from build123d import *

# Parameters (mm, degrees)
BOSS_EXTRUDE4_DEPTH = 5
SKETCH6_W           = 70
SKETCH6_H           = 70
BOSS_EXTRUDE5_DEPTH = 30
SKETCH8_R           = 3
CUT_EXTRUDE1_DEPTH  = 2
FILLET1_R           = 10
CUT_EXTRUDE2_DEPTH  = 30
BOSS_EXTRUDE6_DEPTH = 2.5
SKETCH11_W          = 2.5
SKETCH11_H          = 65
BOSS_EXTRUDE7_DEPTH = 27.5
FILLET2_R           = 10
CHAMFER1_SIZE       = 1.25
CHAMFER2_SIZE       = 1.25


with BuildPart() as part:
    # Sketch5 → Boss-Extrude4 (new body)
    with BuildSketch(Plane(origin=(0, 0, 0), x_dir=(1, 0, 0), z_dir=(0, 1, 0))):
        with BuildLine():
            Line((-22.5, -32.5), (22.5, -32.5))
            ThreePointArc((22.5, -32.5), (29.571067812, -29.571067812), (32.5, -22.5))
            Line((32.5, -22.5), (32.5, 22.5))
            ThreePointArc((32.5, 22.5), (29.571067812, 29.571067812), (22.5, 32.5))
            Line((22.5, 32.5), (-22.5, 32.5))
            ThreePointArc((-22.5, 32.5), (-29.571067812, 29.571067812), (-32.5, 22.5))
            Line((-32.5, 22.5), (-32.5, -22.5))
            ThreePointArc((-32.5, -22.5), (-29.571067812, -29.571067812), (-22.5, -32.5))
        make_face()
    extrude(amount=BOSS_EXTRUDE4_DEPTH)

    # Sketch6 → Boss-Extrude5 (add)
    with BuildSketch(Plane(origin=(0, 5, 0), x_dir=(1, 0, 0), z_dir=(0, 1, 0))):
        Rectangle(SKETCH6_W, SKETCH6_H)
    extrude(amount=BOSS_EXTRUDE5_DEPTH)

    # Sketch8 → Cut-Extrude1 (cut)
    with BuildSketch(Plane.XZ):
        with Locations(Location((26.037533906, -26.035533906, 0), (0, 0, 270))):
            Circle(SKETCH8_R)
        with Locations(Location((26.036533906, 26.036533906, 0), (0, 0, 270))):
            Circle(SKETCH8_R)
        with BuildLine():
            ThreePointArc((-23.035533906, 26.035533906), (-24.887483609, 28.807172503), (-28.156854249, 28.156854249))
            Line((-28.156854249, 28.156854249), (-23.914213562, 23.914213562))
            ThreePointArc((-23.914213562, 23.914213562), (-23.263895308, 24.887483609), (-23.035533906, 26.035533906))
        make_face()
        with BuildLine():
            Line((-23.914213562, 23.914213562), (-28.156854249, 28.156854249))
            ThreePointArc((-28.156854249, 28.156854249), (-28.156854249, 23.914213562), (-23.914213562, 23.914213562))
        make_face()
        with Locations(Location((-26.034533906, -26.036533906, 0), (0, 0, 270))):
            Circle(SKETCH8_R)
    extrude(amount=-CUT_EXTRUDE1_DEPTH, mode=Mode.SUBTRACT)

    # Fillet1
    fillet1_edges = [part.edges().sort_by_distance(p)[0] for p in [
        (-35, 20, -35),
        (-35, 20, 35),
        (35, 20, 35),
        (35, 20, -35),
    ]]
    fillet(fillet1_edges, radius=FILLET1_R)

    # Sketch9 → Cut-Extrude2 (cut)
    with BuildSketch(Plane(origin=(0, 35, 0), x_dir=(1, 0, 0), z_dir=(0, 1, 0))):
        with BuildLine():
            Line((25, 32.5), (-25, 32.5))
            ThreePointArc((-25, 32.5), (-30.303300859, 30.303300859), (-32.5, 25))
            Line((-32.5, 25), (-32.5, -25))
            ThreePointArc((-32.5, -25), (-30.303300859, -30.303300859), (-25, -32.5))
            Line((-25, -32.5), (25, -32.5))
            ThreePointArc((25, -32.5), (30.303300859, -30.303300859), (32.5, -25))
            Line((32.5, -25), (32.5, 25))
            ThreePointArc((32.5, 25), (30.303300859, 30.303300859), (25, 32.5))
        make_face()
    extrude(amount=-CUT_EXTRUDE2_DEPTH, mode=Mode.SUBTRACT)


with BuildPart() as cut_extrude2_piece_1:
    # of the separate pieces the step leaves, piece 1, a body of its own (cut_extrude2_pieces)
    add(part.part.solids().sort_by_distance((-22.5, 0, 32.5))[0])



with BuildPart() as cut_extrude2_piece_2:
    # of the separate pieces the step leaves, piece 2, a body of its own (cut_extrude2_pieces)
    add(part.part.solids().sort_by_distance((25, 5, -35))[0])


with BuildPart() as cut_extrude2_piece_1_1:
    add(cut_extrude2_piece_1.part)

    add(cut_extrude2_piece_2.part)  # Boss-Extrude6 merges Cut-Extrude2 piece 2
    # Sketch10 → Boss-Extrude6 (add)
    with BuildSketch(Plane.XZ.offset(-5)):
        with BuildLine():
            Line((-35, 25), (-35, -25))
            ThreePointArc((-35, -25), (-32.071067812, -32.071067812), (-25, -35))
            Line((-25, -35), (25, -35))
            ThreePointArc((25, -35), (32.071067812, -32.071067812), (35, -25))
            Line((35, -25), (35, 25))
            ThreePointArc((35, 25), (32.071067812, 32.071067812), (25, 35))
            Line((25, 35), (-25, 35))
            ThreePointArc((-25, 35), (-32.071067812, 32.071067812), (-35, 25))
        make_face()
    extrude(amount=-BOSS_EXTRUDE6_DEPTH)

    # Sketch11 → Boss-Extrude7 (add)
    with BuildSketch(Plane(origin=(0, 35, 0), x_dir=(1, 0, 0), z_dir=(0, 1, 0))):
        Rectangle(SKETCH11_W, SKETCH11_H)
    extrude(amount=-BOSS_EXTRUDE7_DEPTH)

    # Fillet2
    fillet2_edges = [cut_extrude2_piece_1_1.edges().sort_by_distance(p)[0] for p in [
        (-1.25, 21.25, -32.5),
        (-1.25, 21.25, 32.5),
        (1.25, 21.25, 32.5),
        (1.25, 21.25, -32.5),
    ]]
    fillet(fillet2_edges, radius=FILLET2_R)

    # Chamfer1
    chamfer1_edges = [cut_extrude2_piece_1_1.edges().sort_by_distance(p)[0] for p in [
        (18.125, 35, -32.5),
        (-30.303300859, 35, -30.303300859),
        (-32.5, 35, 0),
        (-30.303300859, 35, 30.303300859),
        (-18.125, 35, 32.5),
        (30.303300859, 35, 30.303300859),
        (32.5, 35, 0),
        (1.25, 35, 0),
        (18.125, 35, 32.5),
        (-1.25, 35, 0),
        (-18.125, 35, -32.5),
        (4.178932188, 35, -29.571067812),
        (4.178932188, 35, 29.571067812),
        (-4.178932188, 35, 29.571067812),
        (-4.178932188, 35, -29.571067812),
        (30.303300859, 35, -30.303300859),
    ]]
    chamfer(chamfer1_edges, length=CHAMFER1_SIZE - 0.0001)  # a hair under: the kernel refuses the full size

    # Chamfer2
    chamfer2_edges = [cut_extrude2_piece_1_1.edges().sort_by_distance(p)[0] for p in [
        (-29.571067812, 0, 29.571067812),
        (0, 0, 32.5),
        (29.571067812, 0, 29.571067812),
        (32.5, 0, 0),
        (29.571067812, 0, -29.571067812),
        (0, 0, -32.5),
        (-29.571067812, 0, -29.571067812),
        (-32.5, 0, 0),
        (-35, 5, 0),
        (0, 5, -35),
        (35, 5, 0),
        (0, 5, 35),
        (32.071067812, 5, -32.071067812),
        (32.071067812, 5, 32.071067812),
        (-32.071067812, 5, 32.071067812),
        (-32.071067812, 5, -32.071067812),
    ]]
    chamfer(chamfer2_edges, length=CHAMFER2_SIZE)


solid = cut_extrude2_piece_1_1.part
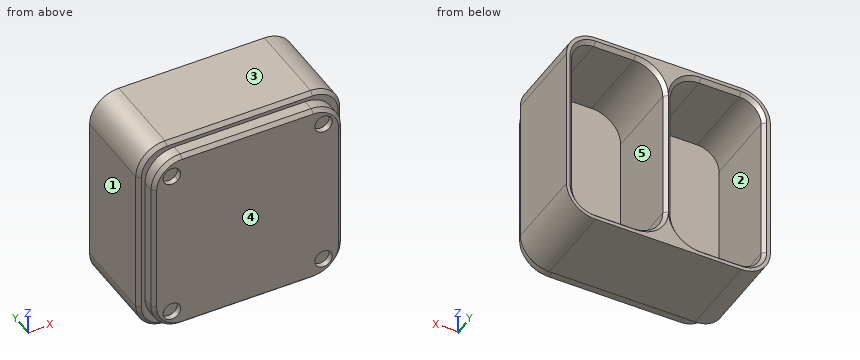
Could you check a few things on this model? Use its own coordinates, in mm. Face numbers are marked on the shaded views. A direction names the side the tool comes from. Coordinates: 2 decimals unless noted, no trailing zeros. Write each loop counter-clockwise with the first axis right and the second up, starting at its lowest first coordinate (ties: lowest second). Pieces come first, ordered by that corner, then holes. Notation, with made-up numbers: M 40,83.5 L 55,83.5 A23 ccw 55,99.5 Z; hole C 39.5,54.5 d7. An arc over 180 degrees is marked long. One line per question, with ' | ' between items.
1) Imagine slicing it at A-A, the plane x = 14.5. Write out the boundary of the cut face in (y, z), and give its area (3 significant figures).
Checks:
outline: M 0,-31.25 L 1.25,-32.5 L 5,-32.5 L 5,-33.75 L 6.25,-35 L 35,-35 L 35,-33.75 L 33.75,-32.5 L 7.5,-32.5 L 7.5,32.5 L 33.75,32.5 L 35,33.75 L 35,35 L 6.25,35 L 5,33.75 L 5,32.5 L 1.25,32.5 L 0,31.25 Z | area: 633 mm²
2) I need wall thicknesses on probe 1 along X at (y, z) = (33.5, 1); probe 2 along Z at (x, y) = (-24, 21.5); probe 3 along X at (y, z) = (14, 31). Which ranges of each line are inside material? Lowest first, please. Write a range as [from, to].
Checks:
probe 1: [-35, -32.5], [-1.25, 1.25], [32.5, 35] | probe 2: [-35, -32.5], [32.5, 35] | probe 3: [-33, -29.5], [-5.98, 5.98], [29.5, 33]
3) If we mould it in two halves opening along Z, with no side actions, what happens to the marked faces 1, 2 and 3? For each: released by +Z, released by -Z, zero draft, split by the parting line, or undercut.
Checks:
face 1: zero draft | face 2: undercut | face 3: released by +Z
4) Imagine slicing it at C-C, the plane y = 20. Write out the boundary of the cut face in (x, z).
Checks:
outline: M -35,-25 A10 ccw -25,-35 L 25,-35 A10 ccw 35,-25 L 35,25 A10 ccw 25,35 L -25,35 A10 ccw -35,25 Z; hole M -32.5,-25 A7.5 ccw -25,-32.5 L -11.25,-32.5 A10 ccw -1.25,-22.5 L -1.25,22.5 A10 ccw -11.25,32.5 L -25,32.5 A7.5 ccw -32.5,25 Z; hole M 1.25,-22.5 A10 ccw 11.25,-32.5 L 25,-32.5 A7.5 ccw 32.5,-25 L 32.5,25 A7.5 ccw 25,32.5 L 11.25,32.5 A10 ccw 1.25,22.5 Z
5) For pin 1 Ø4 at (x, y) = (4, 2.5) entering from -Z; pin 2 Ø8 at (x, z) = (-4, -8.5) entering from -Y; pin 3 Ø8 at (x, z) = (-23, 14) entering from +Y; pin 4 Ø1.8 at (x, z) = (-24.5, 27) entering from -Y, each with a flat end and sliding along its axis, tell me the tip position at first contact or that it passes through.
Checks:
pin 1: z = -32.5 | pin 2: y = 0 | pin 3: y = 7.5 | pin 4: y = 2
6) For the marked faces 4 and 5, which set-ups out of +Z, -Z, +X, -X, +Y, -Y let a thin tool reach every point of the face, with its end or its side?
Checks:
face 4: +Z, -Z, +X, -X, -Y | face 5: +Y
